Could you check a few things on this model? Use its own coordinates, in mm. A direction names the side the tool comes from. Round coordinates to 2 decimals unless told otherwise and drop trailing zeros. Loops run counter-clockwise (first coordinate to the right, second up) from the corner with the lowest first, then second, coordinate; pieces in that order, holes last. Notation, with made-up numbers: (78.5, 32) -> (125.5, 32) arc R23 cw to (125.5, 48) -> close; hole circle Ø9 at (54, 35). An arc over 180 degrees is marked (long way). One line per item, written item: value.
Autodesk Inventor part; units mm, degrees
ref_plane "YZ Plane" through (0, 0, 0) normal (1, 0, 0) x (0, 1, 0)
ref_plane "XZ Plane" through (0, 0, 0) normal (0, 1, 0) x (-1, 0, 0)
ref_plane "XY Plane" through (0, 0, 0) normal (0, 0, 1) x (1, 0, 0)
sketch "Sketch1" plane through (0, 0, 0) normal (0, 1, 0) x (-1, 0, 0)
  line L0 (0, 0) -> (-102, 0)
  line L1 (-102, 0) -> (-102, -4)
  line L2 (-102, -4) -> (0, -4)
  line L3 (0, -4) -> (0, 0)
  line L4 (-102, 0) -> (-98, 0)
  line L5 (-98, 0) -> (-98, -102)
  line L6 (-98, -102) -> (-102, -102)
  line L7 (-102, -102) -> (-102, 0)
  point P0 (-98, -4)
  dimension "d0" = 102
  dimension "d1" = 4
  dimension "d2" = 102
  dimension "d3" = 4
extrude "Extrusion1" add sketch "Sketch1" along normal blind 22.5
sketch "Sketch2" plane through (102, 0, 0) normal (1, 0, 0) x (0, 0, -1)
  line L0 (102, 0) -> (102, 22.5)
  line L1 (102, 11.25) -> (96, 11.25) construction
  circle A0 centre (92.425, 11.25) radius 3.575
  line L2 (88.85, 11.25) -> (28.85, 11.25) construction
  circle A1 centre (25.275, 11.25) radius 3.575
  line L3 (0, 0) -> (0, 22.5)
  line L4 (0, 22.5) -> (102, 22.5)
  point P0 (0, 11.25)
  dimension "d9" = 7.15
  dimension "d6" = 6
  dimension "d7" = 7.15
  dimension "d8" = 60
  dimension "d29" = 25.275
  dimension "d30" = 11.25
sketch "Sketch3" plane through (0, 0, 0) normal (0, 0, 1) x (1, 0, 0)
  line L0 (102, 0) -> (102, 22.5)
  circle A0 centre (76.725, 11.25) radius 3.575
  line L1 (73.15, 11.25) -> (13.15, 11.25)
  circle A1 centre (9.575, 11.25) radius 3.575
  line L2 (0, 11.25) -> (6, 11.25)
  point P0 (0, 0)
  dimension "d11" = 7.15
  dimension "d12" = 60
  dimension "d13" = 7.15
  dimension "d28" = 6
hole "Hole1" at (102, 11.25, -92.425) at (102, 11.25, -25.275) direction (-1, 0, 0) diameter 7.5 depth 10
hole "Hole2" at (9.575, 11.25, 0) at (76.725, 11.25, 0) direction (0, 0, -1) diameter 7.5 depth 10
properties part number "Lbracket"
(1) On a 3-axis mill with a long thin cutter (end or side, diameter ignored), from which of +Z, -Z, +X, -X, +Y, -Y can I reach the whole of each face in a straight line? I mean faces 5 (the face through (50, 11, -4)), 6 (the face through (100, 11, -102)). Say none if no direction works.
Results below:
face 5: -Z, -X, +Y, -Y
face 6: -Z, +X, -X, +Y, -Y
(2) Please list where these lines run through material, in increasing order: L1, parallel to X at y = 11.25, z = -3.1 (3 decimals); L2, parallel to X at y = 16, z = -25; L3, parallel to Z at x = 7, y = 18.5.
Results below:
L1: x = 0 to 5.825, 13.325 to 72.975, 80.475 to 102
L2: x = 98 to 102
L3: z = -4 to 0
(3) We'd pull the mould along X, two halves only. Please class faces 1 (the face through (80.386, 12.063, -2.028)), 2 (the face through (99.97, 10.12, -28.85)), 3 (the face through (98, 11, -52)), 4 (the face through (102, 11, -50)): +X half, -X half, draft (parallel to the pull), parting line (faces both ways), or undercut.
Results below:
face 1: undercut
face 2: draft
face 3: -X half
face 4: +X half
(4) Imagine slicing it at C-C on y = 21.25. Write out the boundary of the cut face in (x, z).
Results below:
outline: (0, -4) -> (98, -4) -> (98, -102) -> (102, -102) -> (102, 0) -> (0, 0) -> close
(5) Imagine slicing it at A-A on y = 11.25. Write out the boundary of the cut face in (x, z) (3 decimals), then the cut area to 3 significant figures.
Results below:
outline: (0, -4) -> (5.825, -4) -> (5.825, 0) -> (0, 0) -> close; (13.325, -4) -> (72.975, -4) -> (72.975, 0) -> (13.325, 0) -> close; (80.475, -4) -> (98, -4) -> (98, -21.525) -> (102, -21.525) -> (102, 0) -> (80.475, 0) -> close; (98, -102) -> (102, -102) -> (102, -96.175) -> (98, -96.175) -> close; (98, -88.675) -> (102, -88.675) -> (102, -29.025) -> (98, -29.025) -> close
area: 680 mm²
(6) For pin 1 Ø5 at (x, y) = (81.5, 17) entering from -Z; pin 2 Ø12 at (y, z) = (11.25, -92.425) entering from -X; pin 3 Ø1 at (x, y) = (22.5, 11) entering from +Z, each with a flat end and sliding along its axis, tell me the tip position at first contact or that it passes through.
Results below:
pin 1: stops at z = -4
pin 2: stops at x = 98
pin 3: stops at z = 0
(7) Imagine slicing it at D-D on x = 24.5. Write out the boundary of the cut face in (y, z), then the cut area to 3 significant figures.
Results below:
outline: (0, -4) -> (22.5, -4) -> (22.5, 0) -> (0, 0) -> close
area: 90.0 mm²
(8) Imagine slicing it at B-B on z = -90.5. Write out the boundary of the cut face in (x, y).
Results below:
outline: (98, 0) -> (102, 0) -> (102, 8.03) -> (98, 8.03) -> close; (98, 14.47) -> (102, 14.47) -> (102, 22.5) -> (98, 22.5) -> close
